Build history of the part. All positions in model axes, mm. Coordinates: 2 decimals unless noted, no trailing zeros. Order: outer loops, then holes, each group sorted by start corner. A loop starts at its lowest first (then second) coordinate and runs counter-clockwise, first axis right, second up. Notation, with made-up numbers: (-4.75, 65) - (52.25, 65) arc R16 ccw to (52.25, 90) - close; hole circle Ø10 at (52.25, 58). An arc over 180 degrees is marked (long way). Write each question's results on one line, items separated by ' | '.
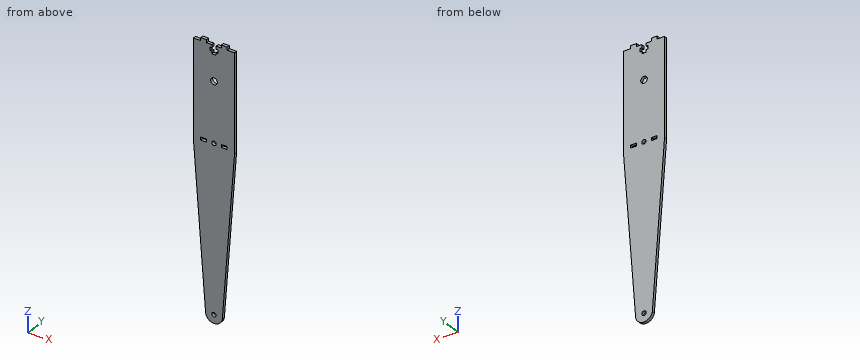
from build123d import *

# Parameters (mm, degrees)
SKETCH1_R           = 1.5
SKETCH1_R_2         = 2.25
SKETCH1_W           = 4
SKETCH1_H           = 2
BOSS_EXTRUDE1_DEPTH = 2
BOSS_EXTRUDE2_DEPTH = 2
SKETCH3_R           = 1.5
CUT_EXTRUDE1_DEPTH  = 2


with BuildPart() as part:
    # Sketch1 → Boss-Extrude1 (new body)
    with BuildSketch(Plane(origin=(0, 0, 0), x_dir=(1, 0, 0), z_dir=(0, 1, 0))):
        Polygon((0, 0), (5, 0), (5, -2), (9, -2), (9, 0), (12.5, 0), (12.5, 2), (11.4, 2), (11.4, 4.3), (12.5, 4.3), (12.5, 6), (15.5, 6), (15.5, 4.3), (16.6, 4.3), (16.6, 2), (15.5, 2), (15.5, 0), (19, 0), (19, -2), (23, -2), (23, 0), (28, 0), (28, 66), (0, 66), align=None)
        with Locations(Location((14, 64, 0), (0, 0, 270))):
            Circle(SKETCH1_R, mode=Mode.SUBTRACT)
        with Locations(Location((14, 23.49, 0), (0, 0, 270))):
            Circle(SKETCH1_R_2, mode=Mode.SUBTRACT)
        with Locations((7, 64)):
            Rectangle(SKETCH1_W, SKETCH1_H, mode=Mode.SUBTRACT)
        with Locations((21, 64)):
            Rectangle(SKETCH1_W, SKETCH1_H, mode=Mode.SUBTRACT)
    extrude(amount=BOSS_EXTRUDE1_DEPTH)

    # Sketch2 → Boss-Extrude2 (add)
    with BuildSketch(Plane(origin=(0, 2, 0), x_dir=(1, 0, 0), z_dir=(0, 1, 0))):
        with BuildLine():
            Line((28, 66), (0, 66))
            Line((0, 66), (9, 186))
            ThreePointArc((9, 186), (14, 191), (19, 186))
            Line((19, 186), (28, 66))
        make_face()
    extrude(amount=-BOSS_EXTRUDE2_DEPTH)

    # Sketch3 → Cut-Extrude1 (cut)
    with BuildSketch(Plane(origin=(0, 2, 0), x_dir=(1, 0, 0), z_dir=(0, 1, 0))):
        with Locations(Location((14, 176, 0), (0, 0, 270))):
            Circle(SKETCH3_R)
        with BuildLine():
            Line((19.75, 176), (22.006411719, 176))
            Line((22.006411719, 176), (22.006411719, 202.106155701))
            Line((22.006411719, 202.106155701), (5.130827786, 202.106155701))
            Line((5.130827786, 202.106155701), (5.130827786, 176))
            Line((5.130827786, 176), (8.25, 176))
            ThreePointArc((8.25, 176), (14, 181.75), (19.75, 176))
        make_face()
    extrude(amount=-CUT_EXTRUDE1_DEPTH, mode=Mode.SUBTRACT)


solid = part.part
1. Band-saw the part on D-D on z = -123. Give the cut face in (x, y) (3 decimals).
Solved:
outline: (4.275, 0) - (23.725, 0) - (23.725, 2) - (4.275, 2) - close
2. Band-saw the part on C-C on y = 1.15. Give the number of separate pieces and of enclosed holes in the cut face, then the cut area to 3 significant figures.
Solved:
separate pieces: 1 | enclosed holes: 5 | area: 4,020 mm2
3. Drop flat-ended pins along their axis: pin 1 Ø1 at (y, z) = (1, 1.5) entering from +X; pin 2 Ø0.6 at (y, z) = (0.5, -1) entering from -X; pin 3 Ø0.9 at (x, y) = (16, 1) entering from -Z; pin 4 Ø1.2 at (x, y) = (12, 1.5) entering from -Z. Give the stop position or say it passes through.
Solved:
pin 1: stops at x = 23 | pin 2: stops at x = 0 | pin 3: stops at z = -181.54 | pin 4: stops at z = -181.58
4. Band-saw the part on A-A on z = -23.49. Give the cut face in (x, y).
Solved:
outline: (0, 0) - (11.75, 0) - (11.75, 2) - (0, 2) - close; (16.25, 0) - (28, 0) - (28, 2) - (16.25, 2) - close
5. Probe line 1 (X direction, y = 1, z = -64); line 2 (Z direction, x = 11.5, y = 1.7); line 3 (X direction, y = 0.55, z = -176). List the from-to ranges inside material, lowest first.
Solved:
line 1: x = 0 to 5, 9 to 12.5, 15.5 to 19, 23 to 28 | line 2: z = -181.18 to -4.3, -2 to 0 | line 3: x = 8.25 to 12.5, 15.5 to 19.75
6. Band-saw the part on B-B on x = 14. Give the cut face in (y, z).
Solved:
outline: (0, -181.75) - (2, -181.75) - (2, -177.5) - (0, -177.5) - close; (0, -174.5) - (2, -174.5) - (2, -65.5) - (0, -65.5) - close; (0, -62.5) - (2, -62.5) - (2, -25.74) - (0, -25.74) - close; (0, -21.24) - (2, -21.24) - (2, -6) - (0, -6) - close
